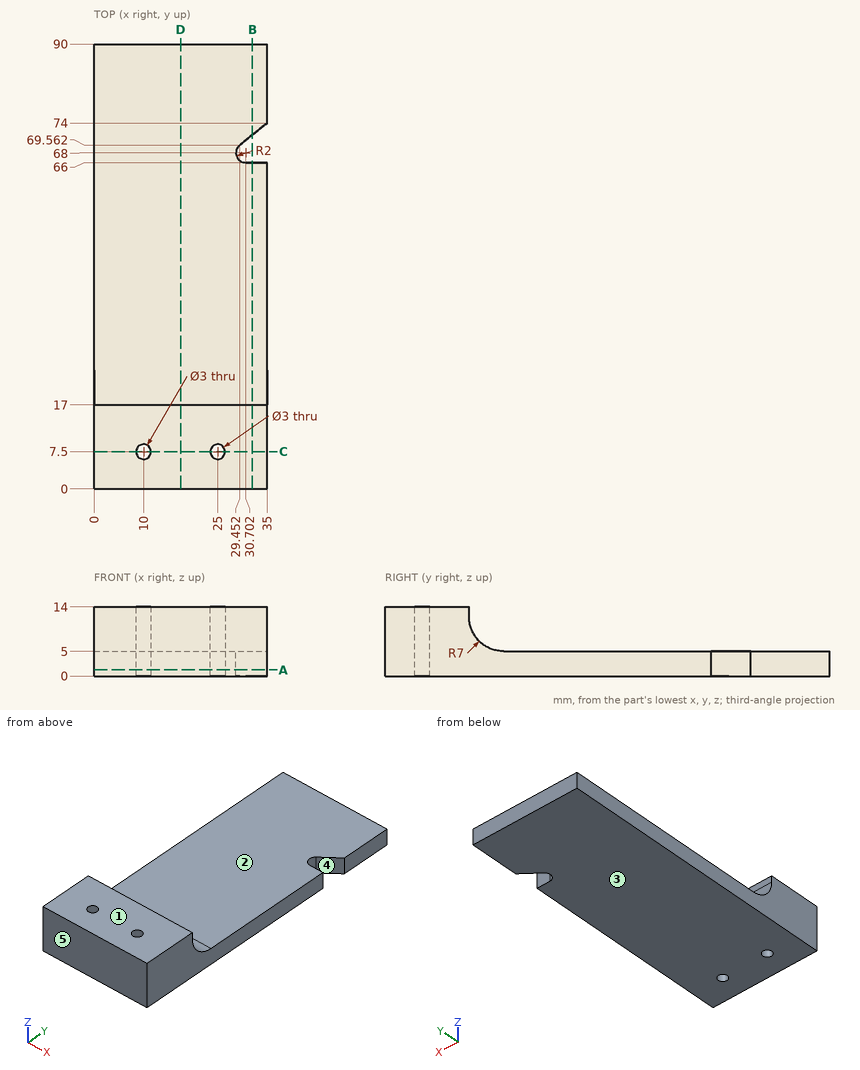
Answer from the drawing. Dimensions are ordinates in mm from the lowest x, y and z of the part. A direction names the side the tool comes from. Give positions to 0.01 mm unless a question says otherwise; leave off trailing zeros. Loops run counter-clockwise (first coordinate to the right, second up) from the corner with the lowest first, then second, coordinate; pieces in that order, holes last.
Item 1: The part is cut by section A-A (z = 1.25). Write down the section's boundary in (x, y).
Item 2: The part is cut by section B-B (x = 32). Write down the section's boundary in (y, z).
Item 3: Find the intervals of material crossed by line 1 along Y through (x, z) = (25, 4); line 2 along Z through (x, y) = (13.5, 25.5); line 3 along Y through (x, z) = (26, 2.25), in increasing order.
Item 4: The mould has two halves that part along Y. Classify the marked faces 3, 4 and 5: released by +Y, released by -Y, zero draft, split by the parting line, or undercut.
Item 5: The part is cut by section C-C (y = 7.5). Write down the section's boundary in (x, z), and give its area (3 significant figures).
Item 6: For the marked faces 1 and 2, determine the directions among +Z, -Z, +X, -X, +Y, -Y from which every point of the face is accessible in a straight line to the end or side of a thin tool.
Item 7: The part is cut by section D-D (x = 17.5). Write down the section's boundary in (y, z).
Item 8: Each of these flat-tipped pins is pushed along its axis until it touches: pin 1 Ø5 at (x, z) = (12.5, 4.5) entering from -Y; pin 2 Ø4 at (x, y) = (23.5, 72) entering from +Z; pin 3 Ø4 at (x, z) = (12.5, 9) entering from +Y; pin 4 Ø2.5 at (x, y) = (10, 7.5) entering from +Z. Where does it stop, or does it pass through?
Taken from the geometry:
1. outline: (0, 0) - (35, 0) - (35, 66) - (30.7, 66) arc R2 cw to (29.45, 69.56) - (35, 74) - (35, 90) - (0, 90) - close; hole circle Ø3 at (10, 7.5); hole circle Ø3 at (25, 7.5)
2. outline: (0, 0) - (66, 0) - (66, 5) - (24, 5) arc R7 cw to (17, 12) - (17, 14) - (0, 14) - close; (71.6, 0) - (90, 0) - (90, 5) - (71.6, 5) - close
3. line 1: y = 0 to 6, 9 to 90
3. line 2: z = 0 to 5
3. line 3: y = 0 to 6.38, 8.62 to 90
4. face 3: zero draft
4. face 4: undercut
4. face 5: released by -Y
5. outline: (0, 0) - (8.5, 0) - (8.5, 14) - (0, 14) - close; (11.5, 0) - (23.5, 0) - (23.5, 14) - (11.5, 14) - close; (26.5, 0) - (35, 0) - (35, 14) - (26.5, 14) - close
5. area: 406 mm2
6. face 1: +Z, +X, -X, +Y, -Y
6. face 2: +Z, +X, -X, +Y
7. outline: (0, 0) - (90, 0) - (90, 5) - (24, 5) arc R7 cw to (17, 12) - (17, 14) - (0, 14) - close
8. pin 1: stops at y = 0
8. pin 2: stops at z = 5
8. pin 3: stops at y = 19.1
8. pin 4: passes through
